The figure shows three views and two pictorial views of one solid part (mm, origin at its lowest corner). Answer the questions. Give positions to 0.01 mm unless a question says otherwise; leave off trailing zeros. Loops run counter-clockwise (first coordinate to the right, second up) from the corner with the lowest first, then second, coordinate; pieces in that order, holes last. Notation, with made-up numbers: (34, 37) - (77, 37) arc R30 cw to (77, 69) - close; hole circle Ø9 at (54, 2). An arc over 180 degrees is marked (long way). Use CSV: the item, a comma, the result in double quotes.
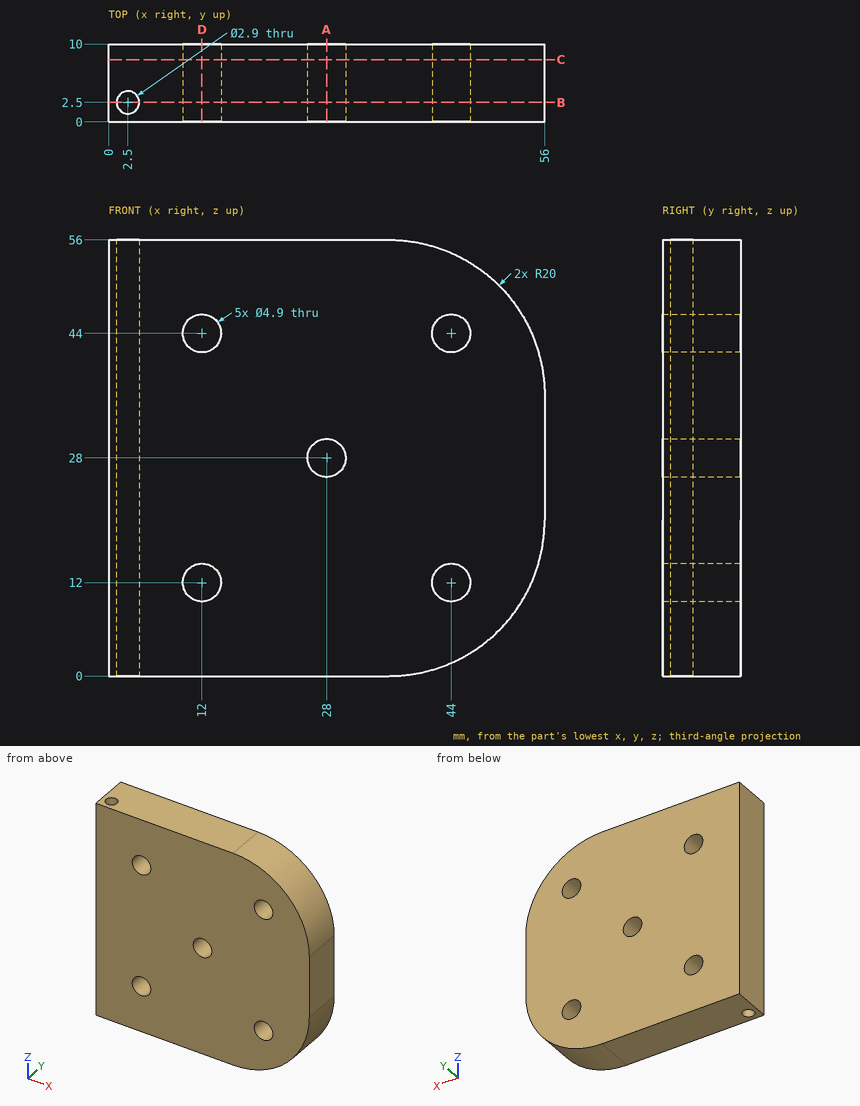
Item 1: A cutting plane is placed at A-A on x = 28. Determine the outline of the cut face in (y, z).
Determined:
outline,"(0, 0) - (10, 0) - (10, 25.55) - (0, 25.55) - close; (0, 30.45) - (10, 30.45) - (10, 56) - (0, 56) - close"
Item 2: A cutting plane is placed at C-C on y = 8. Determine the outline of the cut face in (x, z).
Determined:
outline,"(0, 0) - (36, 0) arc R20 ccw to (56, 20) - (56, 36) arc R20 ccw to (36, 56) - (0, 56) - close; hole circle Ø4.9 at (12, 12); hole circle Ø4.9 at (12, 44); hole circle Ø4.9 at (28, 28); hole circle Ø4.9 at (44, 12); hole circle Ø4.9 at (44, 44)"
Item 3: A cutting plane is placed at B-B on y = 2.5. Determine the outline of the cut face in (x, z).
Determined:
outline,"(0, 0) - (1.05, 0) - (1.05, 56) - (0, 56) - close; (3.95, 0) - (36, 0) arc R20 ccw to (56, 20) - (56, 36) arc R20 ccw to (36, 56) - (3.95, 56) - close; hole circle Ø4.9 at (12, 12); hole circle Ø4.9 at (12, 44); hole circle Ø4.9 at (28, 28); hole circle Ø4.9 at (44, 12); hole circle Ø4.9 at (44, 44)"
Item 4: Given P1, Ø3, axis at x = 44, z = 12, coming from the +Y side, flat-ended and moving along its own axis, determine where the tip first touches the part or whether it passes through.
Determined:
P1,"passes through"
Item 5: A cutting plane is placed at D-D on x = 12. Determine the outline of the cut face in (y, z).
Determined:
outline,"(0, 0) - (10, 0) - (10, 9.55) - (0, 9.55) - close; (0, 14.45) - (10, 14.45) - (10, 41.55) - (0, 41.55) - close; (0, 46.45) - (10, 46.45) - (10, 56) - (0, 56) - close"
Item 6: Find the intervals of material crossed by line 1 (Y direction, x = 2.5, z = 30.5); line 2 (X direction, y = 6, z = 28); line 3 (X direction, y = 3, z = 28), in increasing order.
Determined:
line 1,"y = 0 to 1.05, 3.95 to 10"
line 2,"x = 0 to 25.55, 30.45 to 56"
line 3,"x = 0 to 1.14, 3.86 to 25.55, 30.45 to 56"
